```python
from build123d import *

# Parameters (mm, degrees)
SALIENTE_EXTRUIR1_DEPTH = 40
CROQUIS2_R              = 12.25
SALIENTE_EXTRUIR2_DEPTH = 4
CROQUIS3_R              = 3
CORTAR_EXTRUIR1_DEPTH   = 4


with BuildPart() as part:
    # Croquis1 → Saliente-Extruir1 (new body)
    with BuildSketch(Plane(origin=(0, 0, 0), x_dir=(1, 0, 0), z_dir=(0, 1, 0))):
        with BuildLine():
            Line((-3, 11.87697352), (-3, 8.485281374))
            ThreePointArc((-3, 8.485281374), (0, -9), (3, 8.485281374))
            Line((3, 8.485281374), (3, 11.87697352))
            ThreePointArc((3, 11.87697352), (0, -12.25), (-3, 11.87697352))
        make_face()
    extrude(amount=SALIENTE_EXTRUIR1_DEPTH)

    # Croquis2 → Saliente-Extruir2 (add)
    with BuildSketch(Plane(origin=(0, 40, 0), x_dir=(1, 0, 0), z_dir=(0, 1, 0))):
        with Locations(Location((0, 0, 0), (0, 0, 75.824196484))):
            Circle(CROQUIS2_R)
    extrude(amount=SALIENTE_EXTRUIR2_DEPTH)

    # Croquis3 → Cortar-Extruir1 (cut)
    with BuildSketch(Plane(origin=(0, 44, 0), x_dir=(1, 0, 0), z_dir=(0, 1, 0))):
        with Locations(Location((0, 0, 0), (0, 0, 270))):
            Circle(CROQUIS3_R)
    extrude(amount=-CORTAR_EXTRUIR1_DEPTH, mode=Mode.SUBTRACT)


solid = part.part
```
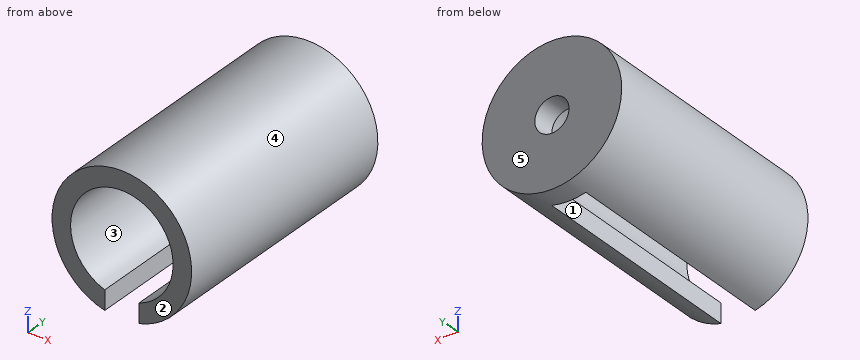
Input: part model. Units: mm. Frame: model coordinates. Face numbers are marked on the shaded views. A direction names the side the tool comes from. Give positions to 0.01 mm unless a question says otherwise; leave off trailing zeros. Loops run counter-clockwise (first coordinate to the right, second up) from the corner with the lowest first, then second, coordinate; pieces in that order, holes last.
1) Contact query for flat-ended pins moving along their axis: pin 1 (4 mm diameter, centred on x = 0, y = 6, fed in from -Z); pin 2 (1 mm diameter, centred on y = 20.5, z = -9.5, fed in from -X); pin 3 (1 mm diameter, centred on y = 12.5, z = -11, fed in from +X). Output: stop coordinate, or through.
A:
pin 1: stops at z = 8.77
pin 2: stops at x = -8.31
pin 3: stops at x = 6.31
2) Section query A-A on x = 0. Return the cut outline in (y, z), and give its area (3 significant figures).
A:
outline: (0, 9) - (40, 9) - (40, 3) - (44, 3) - (44, 12.25) - (0, 12.25) - close; (40, -12.25) - (44, -12.25) - (44, -3) - (40, -3) - close
area: 204 mm2
3) Reachability of the marked faces 1 and 2 from +Z, -Z, +X, -X, +Y, -Y: full face, straight path, thin tool, end or side. Return the list, or none.
A:
face 1: -Z, -Y
face 2: +Z, -Z, +X, -X, -Y
4) Line query: L1, parallel to X at y = 41.1, z = 0; L2, parallel to X at y = 9.5, z = 0; L3, parallel to Y at x = 1.5, z = -7.25. Output: solid intervals per line, ascending.
A:
L1: x = -12.25 to -3, 3 to 12.25
L2: x = -12.25 to -9, 9 to 12.25
L3: y = 40 to 44
5) Section query C-C on y = 38. Return the cut outline in (x, z), and give its area (3 significant figures).
A:
outline: (-3, -11.88) - (-3, -8.49) arc R9 cw (long way) to (3, -8.49) - (3, -11.88) arc R12.25 ccw (long way) to start
area: 197 mm2
6) Mould query, pull axis X, two halves, no side actions, for the marked faces 3, 4 and 5. Classes: released by +X, released by -X, zero draft, split by the parting line, or undercut.
A:
face 3: undercut
face 4: split by the parting line
face 5: zero draft
7) Section query B-B on z = 0. Return the cut outline in (x, y).
A:
outline: (-12.25, 0) - (-9, 0) - (-9, 40) - (-3, 40) - (-3, 44) - (-12.25, 44) - close; (3, 40) - (9, 40) - (9, 0) - (12.25, 0) - (12.25, 44) - (3, 44) - close
8) Section query D-D on z = -10. Return the cut outline in (x, y).
A:
outline: (-7.08, 0) - (-3, 0) - (-3, 40) - (3, 40) - (3, 0) - (7.08, 0) - (7.08, 44) - (-7.08, 44) - close
